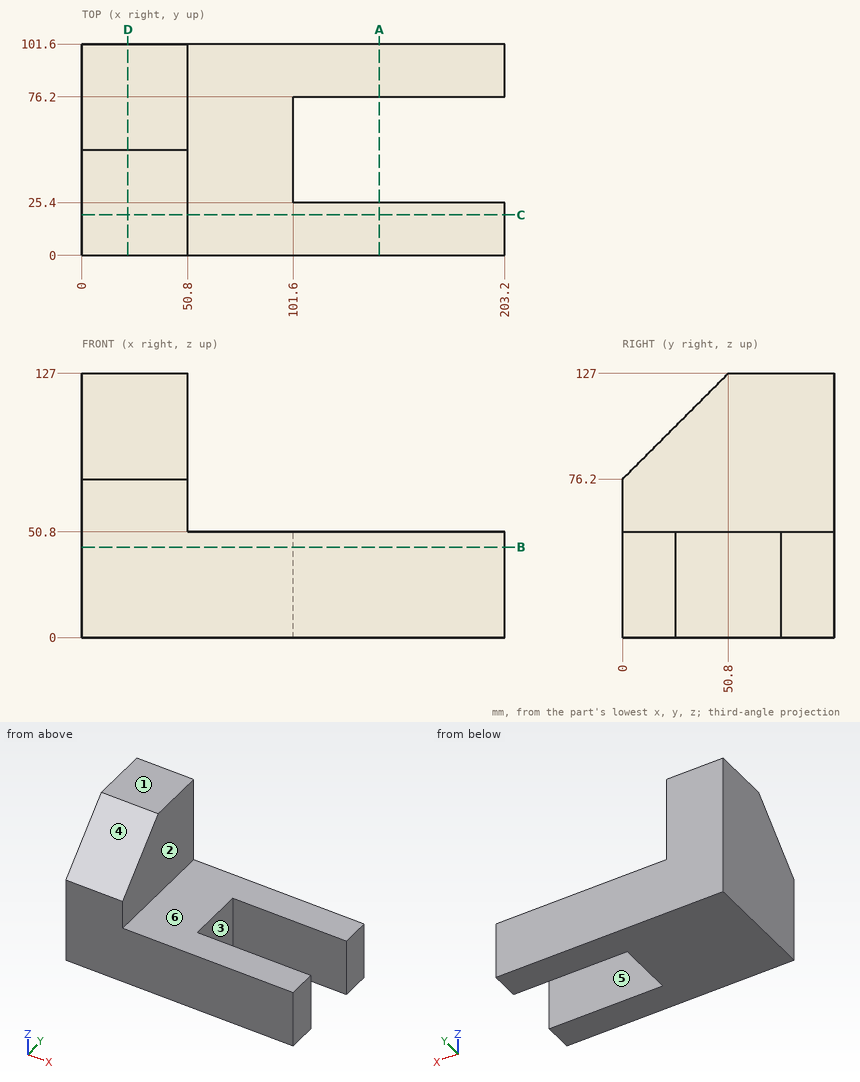
Part print with two shaded views. Sizes in mm from the minimum x, y, z corner. A direction names the side the tool comes from. Round coordinates to 2 decimals unless told otherwise and drop trailing zeros. Order: outer loops, then holes, each group sorted by start corner. A loop starts at its lowest first (then second) coordinate and runs counter-clockwise, first axis right, second up. Notation, with made-up numbers: (53, 30) -> (72, 30) arc R10 cw to (72, 44) -> close; hole circle Ø6 at (-5.5, -8.75). An arc over 180 degrees is marked (long way). Use one line per item in the form item = value.
Item 1: Pull direction Y, two halves, no side cores. Call the marked faces 4, 5 and 6: released by +Y, released by -Y, zero draft, split by the parting line, or undercut.
Returned:
face_4 = released by -Y
face_5 = undercut
face_6 = zero draft
Item 2: Tool access for the marked faces 1, 2 and 3: list every direction of +Z, -Z, +X, -X, +Y, -Y with a clear straight run to the whole face (end or side of a thin tool).
Returned:
face_1 = +Z, +X, -X, +Y, -Y
face_2 = +Z, +X, +Y, -Y
face_3 = +Z, -Z, +X
Item 3: Drill centre lines: line 1 (Y direction, x = 110.5, z = 49); line 2 (Z direction, x = 69, y = 91). Where is each one in solid material? Low to high.
Returned:
line_1 = 0 to 25.4, 76.2 to 101.6
line_2 = 0 to 50.8
Item 4: Cut at B-B, the plane z = 43.5. Write the cut outline in (x, y).
Returned:
outline = (0, 0) -> (203.2, 0) -> (203.2, 25.4) -> (101.6, 25.4) -> (101.6, 76.2) -> (203.2, 76.2) -> (203.2, 101.6) -> (0, 101.6) -> close
Item 5: Cut at A-A, the plane x = 143. Write the cut outline in (y, z), and give its area (3 significant figures).
Returned:
outline = (0, 0) -> (25.4, 0) -> (25.4, 50.8) -> (0, 50.8) -> close; (76.2, 0) -> (101.6, 0) -> (101.6, 50.8) -> (76.2, 50.8) -> close
area = 2,580 mm^2
Item 6: Cut at D-D, the plane x = 22. Write the cut outline in (y, z).
Returned:
outline = (0, 0) -> (101.6, 0) -> (101.6, 127) -> (50.8, 127) -> (0, 76.2) -> close
Item 7: Cut at C-C, the plane y = 19.5. Write the cut outline in (x, z).
Returned:
outline = (0, 0) -> (203.2, 0) -> (203.2, 50.8) -> (50.8, 50.8) -> (50.8, 95.7) -> (0, 95.7) -> close
Item 8: Flat gauge pins, fed straight in: pin 1 Ø1 at (y, z) = (69, 62) entering from +X; pin 2 Ø4 at (y, z) = (50.5, 21) entering from +X; pin 3 Ø3 at (x, y) = (159, 24.5) entering from +Z. Where does each tip first touch, or does it go through?
Returned:
pin_1 = 50.8
pin_2 = 101.6
pin_3 = 50.8
